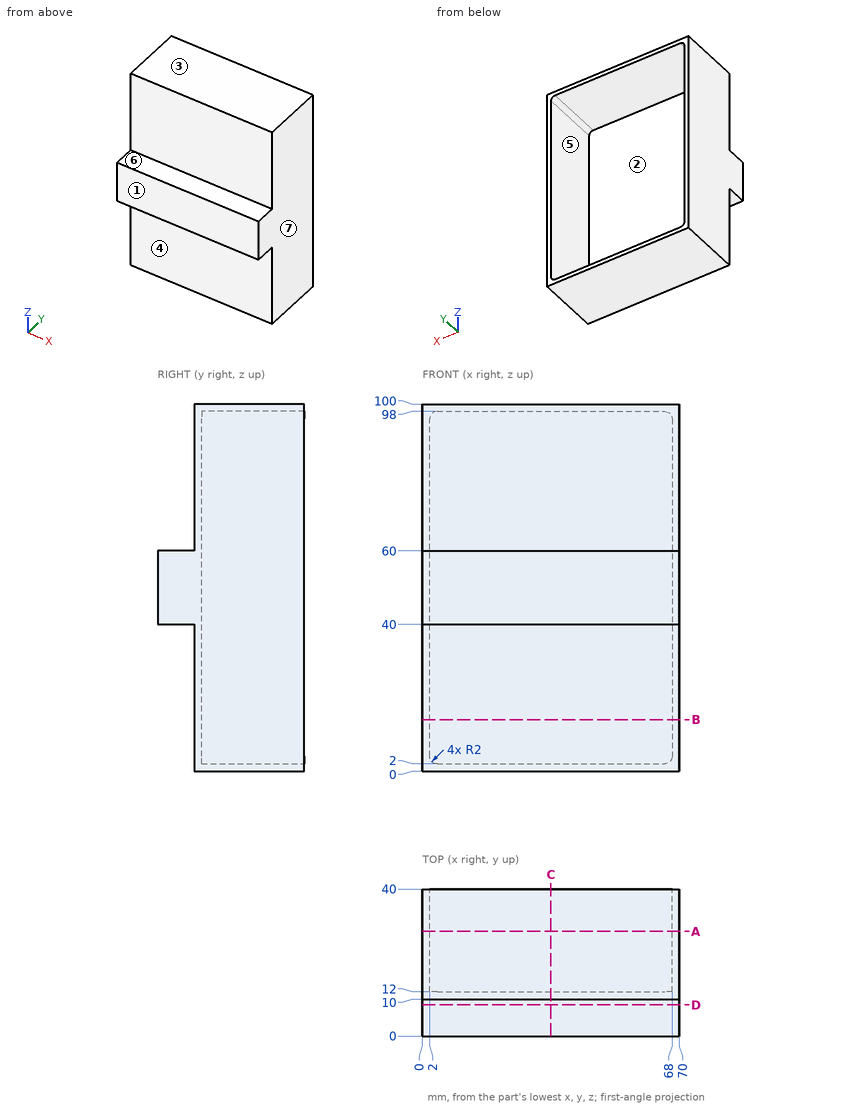
Geometry check sheet. Reference: drawing and pictorial views, mm from the part's lowest x, y, z. A direction names the side the tool comes from. Give positions to 0.01 mm unless a question says otherwise; leave off trailing zeros. Write each loop counter-clockwise with the first axis right and the second up, starting at its lowest first coordinate (ties: lowest second). Pieces come first, ordered by that corner, then holes. Notation, with made-up numbers: M 60,88 L 94,88 A32 ccw 94,116 Z; hole C 62,-11.75 d10. An arc over 180 degrees is marked long. Answer as CSV lines item,"result". Start each with the question number.
Q1. Section check B-B, the plane z = 14. Record the cut outline in (x, y), then the cut area to 3 significant figures.
Q2. Go/stop test with flat-tipped pins: pin 1 (5 mm diameter, centred on x = 49, y = 5.5, fed in from -Z); pin 2 (6 mm diameter, centred on x = 61.5, z = 61.5, fed in from +Y); pin 3 (2 mm diameter, centred on x = 8, z = 32, fed in from -Y). Record where each tip stops, or that it passes through.
Q3. Section check C-C, the plane x = 35. Record the cut outline in (y, z).
Q4. Section check A-A, the plane y = 28.5. Record the cut outline in (x, z), then the cut area to 3 significant figures.
Q5. Material ranges on L1, parallel to X at y = 22.5, z = 12; L2, parallel to Z at x = 11, y = 28; L3, parallel to Y at x = 64.5, z = 93.5, recorded low to high.
Q6. Release check for a two-part mould opening along Z. For the marked faces 1, 2 and 3 record: pulls with the +Z half, pulls with the -Z half, needs draft (parallel to the pull), parting line crosses it, or undercut.
Q7. Section check D-D, the plane y = 8.5. Record the cut outline in (x, z), then the cut area to 3 significant figures.
Q8. Tool access check on the marked faces 4, 5, 6 and 7. Record the directions out of +Z, -Z, +X, -X, +Y, -Y that give a thin tool (end or side, any length) a straight path to the whole face; none if there is none.
Geometry says:
1,outline,"M 0,10 L 70,10 L 70,40 L 68,40 L 68,12 L 2,12 L 2,40 L 0,40 Z"
1,area,"252 mm^2"
2,pin 1,"z = 40"
2,pin 2,"y = 12"
2,pin 3,"y = 10"
3,outline,"M 0,40 L 10,40 L 10,0 L 40,0 L 40,2 L 12,2 L 12,98 L 40,98 L 40,100 L 10,100 L 10,60 L 0,60 Z"
4,outline,"M 0,0 L 70,0 L 70,100 L 0,100 Z; hole M 2,4 A2 ccw 4,2 L 66,2 A2 ccw 68,4 L 68,96 A2 ccw 66,98 L 4,98 A2 ccw 2,96 Z"
4,area,"667 mm^2"
5,L1,"0 to 2, 68 to 70"
5,L2,"0 to 2, 98 to 100"
5,L3,"10 to 12"
6,face 1,"needs draft"
6,face 2,"undercut"
6,face 3,"pulls with the +Z half"
7,outline,"M 0,40 L 70,40 L 70,60 L 0,60 Z"
7,area,"1,400 mm^2"
8,face 4,"-Z, +X, -X, -Y"
8,face 5,"+Y"
8,face 6,"+Z, +X, -X, -Y"
8,face 7,"+Z, -Z, +X, +Y, -Y"
